Work out the finished part from the listing and answer in its coordinate system (mm). Face numbers are marked on the shaded views. A direction names the side the tool comes from. Coordinates: 2 decimals unless noted, no trailing zeros. Write each loop counter-clockwise with the first axis right and the second up, starting at its lowest first coordinate (ties: lowest second). Pieces come first, ordered by that corner, then holes. Notation, with made-up numbers: (-7.75, 81) - (50.25, 81) arc R14 cw to (50.25, 104) - close; hole circle Ø5 at (49, 49.5). An arc over 180 degrees is marked (long way). Use a Markdown table: item, result. Add a question column.
(1) For a pull along Z with two mould halves and no side action, classify the marked faces 5, 6 and 7 as released by +Z, released by -Z, zero draft, split by the parting line, or undercut.
(2) Given pin 1 Ø0.8 at (y, z) = (18, 1.5) entering from +X; pin 2 Ø16 at (x, z) = (-4.5, 7.5) entering from +Y; pin 3 Ø5 at (x, y) = (29.5, 15.5) entering from +Z; pin 4 Ø6.5 at (y, z) = (9, 11) entering from -X, each flat-ended and moving along its own axis, determine where each tip first touches the part or whether it passes through.
(3) Find the intervals of material crossed by line 1 (X direction, y = 11, z = 0); line 2 (Z direction, x = 0, y = 25.3); line 3 (Z direction, x = 0, y = 3), in increasing order. Write a range as from..to.
(4) A tool of negligible diameter and unlimited length cuts with its end or side. For the marked faces 1, 2, 3 and 4, from which of +Z, -Z, +X, -X, +Y, -Y can it reach the whole face along a straight path? Write none if from no direction.
(5) The part is cut by section D-D, the plane x = -20.5. Give the vertices of the cut face in (y, z).
(6) The part is cut by section C-C, the plane x = 39. Give the vertices of the cut face in (y, z), then the cut area to 3 significant figures.
(7) The part is cut by section A-A, the plane x = 0. Give the vertices of the cut face in (y, z).
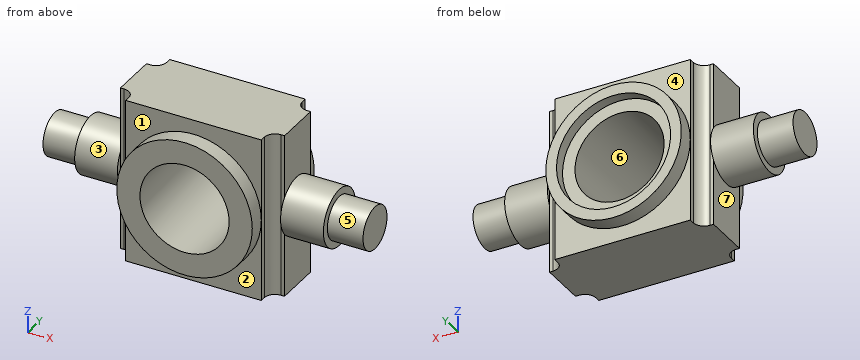
from build123d import *

# Parameters (mm, degrees)
SKETCH1_W           = 46
SKETCH1_H           = 46
BOSS_EXTRUDE1_DEPTH = 22
SKETCH2_R           = 19
BOSS_EXTRUDE4_DEPTH = 4.5
SKETCH5_R           = 19
BOSS_EXTRUDE5_DEPTH = 4.5
SKETCH6_R           = 16
CUT_EXTRUDE1_DEPTH  = 3
SKETCH7_R           = 12.5
CUT_EXTRUDE2_DEPTH  = 29
SKETCH8_R           = 8
BOSS_EXTRUDE6_DEPTH = 12
SKETCH9_R           = 6
BOSS_EXTRUDE7_DEPTH = 10
SKETCH10_R          = 8
BOSS_EXTRUDE8_DEPTH = 12
SKETCH11_R          = 6
BOSS_EXTRUDE9_DEPTH = 10
CUT_EXTRUDE3_DEPTH  = 47


with BuildPart() as part:
    # Sketch1 → Boss-Extrude1 (new body)
    with BuildSketch(Plane(origin=(0, 0, 0), x_dir=(1, 0, 0), z_dir=(0, 1, 0))):
        Rectangle(SKETCH1_W, SKETCH1_H)
    extrude(amount=BOSS_EXTRUDE1_DEPTH)

    # Sketch2 → Boss-Extrude4 (add)
    with BuildSketch(Plane(origin=(0, 22, 0), x_dir=(1, 0, 0), z_dir=(0, 1, 0))):
        Circle(SKETCH2_R)
    extrude(amount=BOSS_EXTRUDE4_DEPTH)

    # Sketch5 → Boss-Extrude5 (add)
    with BuildSketch(Plane.XZ):
        Circle(SKETCH5_R)
    extrude(amount=BOSS_EXTRUDE5_DEPTH)

    # Sketch6 → Cut-Extrude1 (cut)
    with BuildSketch(Plane(origin=(0, 26.5, 0), x_dir=(1, 0, 0), z_dir=(0, 1, 0))):
        Circle(SKETCH6_R)
    extrude(amount=-CUT_EXTRUDE1_DEPTH, mode=Mode.SUBTRACT)

    # Sketch7 → Cut-Extrude2 (cut, through all)
    with BuildSketch(Plane(origin=(0, 23.5, 0), x_dir=(1, 0, 0), z_dir=(0, 1, 0))):
        Circle(SKETCH7_R)
    extrude(amount=-CUT_EXTRUDE2_DEPTH, mode=Mode.SUBTRACT)

    # Sketch8 → Boss-Extrude6 (add)
    with BuildSketch(Plane(origin=(23, 0, 0), x_dir=(0, 0, -1), z_dir=(1, 0, 0))):
        with Locations((0, 10.505702785)):
            Circle(SKETCH8_R)
    extrude(amount=BOSS_EXTRUDE6_DEPTH)

    # Sketch9 → Boss-Extrude7 (add)
    with BuildSketch(Plane(origin=(35, 0, 0), x_dir=(0, 0, -1), z_dir=(1, 0, 0))):
        with Locations((0, 10.505702785)):
            Circle(SKETCH9_R)
    extrude(amount=BOSS_EXTRUDE7_DEPTH)

    # Sketch10 → Boss-Extrude8 (add)
    with BuildSketch(Plane.ZY.offset(23)):
        with Locations((0, 11)):
            Circle(SKETCH10_R)
    extrude(amount=BOSS_EXTRUDE8_DEPTH)

    # Sketch11 → Boss-Extrude9 (add)
    with BuildSketch(Plane.ZY.offset(35)):
        with Locations((0, 11)):
            Circle(SKETCH11_R)
    extrude(amount=BOSS_EXTRUDE9_DEPTH)

    # Sketch13 → Cut-Extrude3 (cut, through all)
    with BuildSketch(Plane.XY.offset(23)):
        with BuildLine():
            Line((-23, 22), (-19, 22))
            Line((-19, 22), (-19, 20.5))
            ThreePointArc((-19, 20.5), (-19.878679656, 18.378679656), (-22, 17.5))
            Line((-22, 17.5), (-23, 17.5))
            Line((-23, 17.5), (-23, 22))
        make_face()
        with BuildLine():
            Line((23, 22), (19, 22))
            Line((19, 22), (19, 20.5))
            ThreePointArc((19, 20.5), (19.878679656, 18.378679656), (22, 17.5))
            Line((22, 17.5), (23, 17.5))
            Line((23, 17.5), (23, 22))
        make_face()
        with BuildLine():
            Line((-23, 0), (-19, 0))
            Line((-19, 0), (-19, 1.5))
            ThreePointArc((-19, 1.5), (-19.878679656, 3.621320344), (-22, 4.5))
            Line((-22, 4.5), (-23, 4.5))
            Line((-23, 4.5), (-23, 0))
        make_face()
        with BuildLine():
            Line((23, 0), (23, 4.5))
            Line((23, 4.5), (22, 4.5))
            ThreePointArc((22, 4.5), (19.878679656, 3.621320344), (19, 1.5))
            Line((19, 1.5), (19, 0))
            Line((19, 0), (23, 0))
        make_face()
    extrude(amount=-CUT_EXTRUDE3_DEPTH, mode=Mode.SUBTRACT)


solid = part.part
Model answer:
| question | item | result |
|---|---|---|
| 1 | face 5 | split by the parting line |
| 1 | face 6 | undercut |
| 1 | face 7 | zero draft |
| 2 | pin 1 | x = 35 |
| 2 | pin 2 | y = 26.5 |
| 2 | pin 3 | z = 7.6 |
| 2 | pin 4 | x = -35 |
| 3 | line 1 | -45..-12.5, 12.5..45 |
| 3 | line 2 | -19..-16, 16..19 |
| 3 | line 3 | -23..-12.5, 12.5..23 |
| 4 | face 1 | +Z, -Y |
| 4 | face 2 | -Z, -Y |
| 4 | face 3 | -X |
| 4 | face 4 | +Z, +Y |
| 5 | outline | (4.1, -23) - (17.9, -23) - (17.9, 23) - (4.1, 23) - close |
| 6 | outline | circle Ø12 at (10.51, 0) |
| 6 | area | 113 mm^2 |
| 7 | outline | (-4.5, -19) - (0, -19) - (0, -23) - (22, -23) - (22, -19) - (26.5, -19) - (26.5, -16) - (23.5, -16) - (23.5, -12.5) - (-4.5, -12.5) - close; (-4.5, 12.5) - (23.5, 12.5) - (23.5, 16) - (26.5, 16) - (26.5, 19) - (22, 19) - (22, 23) - (0, 23) - (0, 19) - (-4.5, 19) - close |
